The listing builds one solid part. Answer for the finished solid, in the listing's coordinates (mm). Give positions to 0.01 mm unless a question says otherwise; leave off trailing zeros. Write each loop counter-clockwise with the first axis right and the second up, starting at its lowest first coordinate (ties: lowest second). Pieces come first, ordered by that corner, then holes. Notation, with made-up numbers: (-27.5, 64.5) -> (0.5, 64.5) arc R17 ccw to (0.5, 82.5) -> close; hole circle Ø11 at (64.5, 21). An arc over 180 degrees is marked (long way). Use CSV: the item, a comma, the result in double quotes. Start each with the question number.
Solid Edge part; units mm, degrees
sketch "Sketch1" plane through (0, 0, 0) normal (0, 0, 1) x (1, 0, 0)
  line L0 (6.3, 6.3) -> (6.3, -6.3)
  line L1 (6.3, -6.3) -> (-6.3, -6.3)
  line L2 (-6.3, -6.3) -> (-6.3, 6.3)
  line L3 (-6.3, 6.3) -> (6.3, 6.3)
extrude "Protrusion1" add sketch "Sketch1" along normal blind 5.7
chamfer "Chanfrein_1" distance 2.9 angle 63 4 edges at (0, -6.3, 5.7) (6.3, 0, 5.7) (0, 6.3, 5.7) (-6.3, 0, 5.7) measured on face at (4.326, -4.074, 5.7)
Q1. Straight lines are drawn through the part: L1, parallel to Y at x = -0.25, z = 0.4; L2, parallel to Y at x = 3, z = 0.6; L3, parallel to Z at x = -3.5, y = -4. For each, find the intervals that lie inside material, in ascending order.
Q2. Section D-D on z = 4.95 is taken. Give the vertices of the cut face in (x, y), then the cut area to 3 significant figures.
Q3. Section C-C on z = 3.4 is taken. Give the vertices of the cut face in (x, y), then the cut area to 3 significant figures.
Q4. Flat-ended cylindrical pins translate along their axes: pin 1 Ø1.5 at (x, z) = (-4.5, 4.5) entering from -Y; pin 2 Ø1 at (y, z) = (-3, 5) entering from -X; pin 3 Ø2 at (y, z) = (-4, 4) entering from -X. Find the tip coordinate at first contact, or state that the pin passes through.
Output:
1,L1,"-6.1 to 6.1"
1,L2,"-6 to 6"
1,L3,"0 to 4.52"
2,outline,"(-3.78, -3.78) -> (3.78, -3.78) -> (3.78, 3.78) -> (-3.78, 3.78) -> close"
2,area,"57.2 mm²"
3,outline,"(-4.57, -4.57) -> (4.57, -4.57) -> (4.57, 4.57) -> (-4.57, 4.57) -> close"
3,area,"83.6 mm²"
4,pin 1,"y = -4.39"
4,pin 2,"x = -4.01"
4,pin 3,"x = -4.78"
